from build123d import *

# Parameters (mm, degrees)
SKETCH1_W           = 12.7
SKETCH1_H           = 38.1
SKETCH1_R           = 1.905
BOSS_EXTRUDE1_DEPTH = 180.34
SKETCH3_W           = 167.64
SKETCH3_H           = 12.7
CUT_EXTRUDE1_DEPTH  = 182.787535601
FILLET1_R           = 2.54


with BuildPart() as part:
    # Sketch1 → Boss-Extrude1 (new body)
    with BuildSketch(Plane(origin=(0, 0, 0), x_dir=(0, 0, -1), z_dir=(1, 0, 0))):
        Rectangle(SKETCH1_W, SKETCH1_H)
        with Locations((0, -12.7)):
            Circle(SKETCH1_R, mode=Mode.SUBTRACT)
        with Locations((0, 12.7)):
            Circle(SKETCH1_R, mode=Mode.SUBTRACT)
    extrude(amount=-BOSS_EXTRUDE1_DEPTH)

    # Sketch3 → Cut-Extrude1 (cut, through all)
    with BuildSketch(Plane.XY.offset(6.35)):
        with Locations((-90.17, 0)):
            Rectangle(SKETCH3_W, SKETCH3_H)
    extrude(amount=-CUT_EXTRUDE1_DEPTH, mode=Mode.SUBTRACT)

    # Fillet1
    fillet1_edges = [part.edges().sort_by_distance(p)[0] for p in [
        (-6.35, 0, -6.35),
        (-6.35, 6.35, 0),
        (-90.17, -6.35, -6.35),
        (-6.35, -6.35, 0),
        (-173.99, 0, -6.35),
        (-173.99, -6.35, 0),
        (-90.17, 6.35, -6.35),
        (-173.99, 6.35, 0),
        (-6.35, 0, 6.35),
        (-90.17, 6.35, 6.35),
        (-173.99, 0, 6.35),
        (-90.17, -6.35, 6.35),
        (-90.17, 19.05, 6.35),
        (-90.17, 19.05, -6.35),
        (-90.17, -19.05, -6.35),
        (-90.17, -19.05, 6.35),
    ]]
    fillet(fillet1_edges, radius=FILLET1_R)


solid = part.part
For this review, take the finished solid that the model builds, in its own axes (mm). A direction names the side the tool comes from. Give positions to 0.01 mm unless a question says otherwise; leave off trailing zeros. Loops run counter-clockwise (first coordinate to the right, second up) from the corner with the lowest first, then second, coordinate; pieces in that order, holes last. Notation, with made-up numbers: M 6,-3 L 13,-3 A10 ccw 13,9 Z; hole C 66,-31.5 d4. An arc over 180 degrees is marked long. Answer as a JSON object with one key per item and string values. Group by question number.
Q1. For probe 1 along Y at (x, z) = (-62, 0) (3 decimals); probe 2 along Y at (x, z) = (-135, -3.25); probe 3 along Z at (x, y) = (-81.5, -12.5), list the stretches that pass through material, from the lowest coordinate up. Write a range as [from, to].
Q2. Add section B-B on y = 12.7. Give the boundary of the cut face in (x, z) (3 decimals), and give its area (3 significant figures).
Q3. Add section C-C on z = 0. Give the boundary of the cut face in (x, y) (3 decimals).
Q4. Add section D-D on y = -1. Give the boundary of the cut face in (x, z), and give its area (3 significant figures).
Q5. Mouldability with a two-part tool opening along Z and no side actions: class faces 1 (the flat face through (-180.34, 0, 0)), 2 (the cylindrical face through (-88.91, 10.84, 0.41)), 3 (the cylindrical face through (-88.91, -14.56, 0.41)), 4 (the flat face through (-89, -11, 6.35)) as +Z half, -Z half, draft (parallel to the pull), parting line (faces both ways), or undercut.
Q6. Tool access review of faces 5 (the flat face through (-6.35, 0, 0)), 6 (the flat face through (0, 0, 0)): name each direction out of +Z, -Z, +X, -X, +Y, -Y from which nothing blocks a thin tool from reaching the whole face with its end or side.
Q7. Insertion check: P1, Ø3.5, axis at y = 12.7, z = 0, coming from the -X side. The pin has a flat end and moves straight along its axis. Give the tip position at first contact, or say it passes through.
Q8. Add section A-A on x = -110. Give the boundary of the cut face in (y, z) (3 decimals), and give its area (3 significant figures).
Checked values:
{
 "1": {"probe 1": "[-19.05, -14.605], [-10.795, -6.35], [6.35, 10.795], [14.605, 19.05]", "probe 2": "[-19.05, -6.35], [6.35, 19.05]", "probe 3": "[-6.35, -1.89], [1.89, 6.35]"},
 "2": {"outline": "M -180.34,-6.35 L 0,-6.35 L 0,-1.905 L -180.34,-1.905 Z; M -180.34,1.905 L 0,1.905 L 0,6.35 L -180.34,6.35 Z", "area": "1,600 mm²"},
 "3": {"outline": "M -180.34,-19.05 L 0,-19.05 L 0,-14.605 L -180.34,-14.605 Z; M -180.34,-10.795 L 0,-10.795 L 0,10.795 L -180.34,10.795 Z; M -180.34,14.605 L 0,14.605 L 0,19.05 L -180.34,19.05 Z; hole M -173.99,-3.81 A2.54 ccw -171.45,-6.35 L -8.89,-6.35 A2.54 ccw -6.35,-3.81 L -6.35,3.81 A2.54 ccw -8.89,6.35 L -171.45,6.35 A2.54 ccw -173.99,3.81 Z"},
 "4": {"outline": "M -180.34,-6.35 L -176.53,-6.35 A2.54 ccw -173.99,-3.81 L -173.99,3.81 A2.54 ccw -176.53,6.35 L -180.34,6.35 Z; M -6.35,-3.81 A2.54 ccw -3.81,-6.35 L 0,-6.35 L 0,6.35 L -3.81,6.35 A2.54 ccw -6.35,3.81 Z", "area": "156 mm²"},
 "5": {"face 1": "draft", "face 2": "undercut", "face 3": "undercut", "face 4": "+Z half"},
 "6": {"face 5": "+Z, -Z", "face 6": "+Z, -Z, +X, +Y, -Y"},
 "7": {"P1": "through"},
 "8": {"outline": "M -19.05,-3.81 A2.54 ccw -16.51,-6.35 L -8.89,-6.35 A2.54 ccw -6.35,-3.81 L -6.35,3.81 A2.54 ccw -8.89,6.35 L -16.51,6.35 A2.54 ccw -19.05,3.81 Z; M 6.35,-3.81 A2.54 ccw 8.89,-6.35 L 16.51,-6.35 A2.54 ccw 19.05,-3.81 L 19.05,3.81 A2.54 ccw 16.51,6.35 L 8.89,6.35 A2.54 ccw 6.35,3.81 Z; hole C -12.7,0 d3.81; hole C 12.7,0 d3.81", "area": "289 mm²"}
}
